Check sheet for the modelled part. Datum: model origin and axes. Units: mm. Round coordinates to 2 decimals unless told otherwise and drop trailing zeros. Order: outer loops, then holes, each group sorted by start corner. A loop starts at its lowest first (then second) coordinate and runs counter-clockwise, first axis right, second up.
```python
from build123d import *

# Parameters (mm, degrees)
F0_R     = 37.7825
F1_DEPTH = 12.7
F2_R     = 6.35
F3_R     = 6.34999
F4_R     = 1.4986
F5_DEPTH = 12.701


# Not quite as in the source:
# - a fillet or chamfer is up to 0.001 mm smaller than in the source, because OpenCascade refuses the exact size


with BuildPart() as f1:
    # F0 (on Front) → F1 (new body)
    with BuildSketch(Plane.XZ):
        with Locations((-56.96824193, 43.9220815897)):
            Circle(F0_R)
    extrude(amount=F1_DEPTH)

    # F2
    f2_edges = [f1.edges().sort_by_distance(p)[0] for p in [
        (-94.750742, -12.7, 43.922082),
    ]]
    fillet(f2_edges, radius=F2_R)

    # F3 (radius 6.35 in the source; OpenCascade refuses exactly that, so slightly less here)
    f3_edges = [f1.edges().sort_by_distance(p)[0] for p in [
        (-94.750742, 0, 43.922082),
    ]]
    fillet(f3_edges, radius=F3_R)

    # F4 (on face) → F5 (cut, through all)
    with BuildSketch(Plane.XZ.offset(12.7)):
        with Locations((-56.96824193, 43.9220815897)):
            Circle(F4_R)
    extrude(amount=-F5_DEPTH, mode=Mode.SUBTRACT)


solid = f1.part
```
Item 1: Scan lines: line 1 along Z through (x, y) = (-69.5, -7); line 2 along Z through (x, y) = (-27.5, -2.75); line 3 along Y through (x, z) = (-69, 10.5). Record each from-to range of solid material in increasing order.
Answer:
line 1: z = 8.31 to 79.53
line 2: z = 22.11 to 65.74
line 3: y = -11.21 to -1.49
Item 2: Release check for a two-part mould opening along Z. For faces 1 (the cylindrical face through (-58.073, -6.439, 44.935)), 2 (the flat face through (-57, 0, 37)) record: released by +Z, released by -Z, zero draft, split by the parting line, or undercut.
Answer:
face 1: undercut
face 2: zero draft
Item 3: Sectioned sample at A-A (y = -4.25). Record the cut outline in (x, z).
Answer:
outline: circle Ø74.85 at (-56.97, 43.92); hole circle Ø3 at (-56.97, 43.92)
Item 4: Sectioned sample at B-B (y = -8.25). Record the cut outline in (x, z), and give its area (3 significant figures).
Answer:
outline: circle Ø74.98 at (-56.97, 43.92); hole circle Ø3 at (-56.97, 43.92)
area: 4,410 mm2
Item 5: Go/stop test with flat-tipped pins: P1, Ø4, axis at x = -37.5, y = -10, coming from the -Z side; P2, Ø2, axis at x = -56, y = -8.5, coming from the -Z side. Record where each tip stops, or that it passes through.
Answer:
P1: stops at z = 11.19
P2: stops at z = 6.26
